from build123d import *

# Parameters (mm, degrees)
ESQUISSE1_W        = 39.37
ESQUISSE1_H        = 35.56
ESQUISSE1_R        = 1.65
BOSS_EXTRU_1_DEPTH = 2
CONG_2_R           = 5


with BuildPart() as part:
    # Esquisse1 → Boss.-Extru.1 (new body)
    with BuildSketch(Plane(origin=(0, 0, 0), x_dir=(1, 0, 0), z_dir=(0, 1, 0))):
        Rectangle(ESQUISSE1_W, ESQUISSE1_H)
        with Locations((-15.855, 13.97)):
            Circle(ESQUISSE1_R, mode=Mode.SUBTRACT)
        with Locations((15.855, 13.97)):
            Circle(ESQUISSE1_R, mode=Mode.SUBTRACT)
        with Locations((-15.855, -13.97)):
            Circle(ESQUISSE1_R, mode=Mode.SUBTRACT)
        with Locations((15.855, -13.97)):
            Circle(ESQUISSE1_R, mode=Mode.SUBTRACT)
    extrude(amount=BOSS_EXTRU_1_DEPTH)

    # Congé2
    cong_2_edges = [part.edges().sort_by_distance(p)[0] for p in [
        (19.685, 1, 17.78),
        (-19.685, 1, 17.78),
        (-19.685, 1, -17.78),
        (19.685, 1, -17.78),
    ]]
    fillet(cong_2_edges, radius=CONG_2_R)


solid = part.part
The listing builds one solid part. Answer for the finished solid, in the listing's coordinates (mm). Give positions to 0.01 mm unless a question says otherwise; leave off trailing zeros. Order: outer loops, then holes, each group sorted by start corner. A loop starts at its lowest first (then second) coordinate and runs counter-clockwise, first axis right, second up. Notation, with made-up numbers: (15, 69) - (42, 69) arc R28 ccw to (42, 93) - close; hole circle Ø3 at (40.5, 49.5). An arc over 180 degrees is marked (long way). Use one line per item in the form item = value.
1) The mould has two halves that part along Z. Classify faces 1 (the cylindrical face through (18.181, 1.014, -16.354)), 2 (the flat face through (0, 2, 0)), 3 (the cylindrical face through (-16.21, 0.99, -12.36)): released by +Z, released by -Z, zero draft, split by the parting line, or undercut.
Verdict:
face_1 = released by -Z
face_2 = zero draft
face_3 = undercut
2) Find section A-A on y = 0.3. Determine the outline of the cut face in (x, z) (3 decimals), and give its area (3 significant figures).
Verdict:
outline = (-19.685, -12.78) arc R5 ccw to (-14.685, -17.78) - (14.685, -17.78) arc R5 ccw to (19.685, -12.78) - (19.685, 12.78) arc R5 ccw to (14.685, 17.78) - (-14.685, 17.78) arc R5 ccw to (-19.685, 12.78) - close; hole circle Ø3.3 at (-15.855, -13.97); hole circle Ø3.3 at (-15.855, 13.97); hole circle Ø3.3 at (15.855, -13.97); hole circle Ø3.3 at (15.855, 13.97)
area = 1,340 mm^2
3) This flat-tipped pin is pushed along its axis until it touches: pin 1 (3 mm diameter, centred on x = 15.855, z = -13.97, fed in from -Y). Where does it stop, or does it pass through?
Verdict:
pin_1 = through
4) Find section C-C on x = -16. Determine the outline of the cut face in (y, z).
Verdict:
outline = (0, -17.6) - (2, -17.6) - (2, -15.61) - (0, -15.61) - close; (0, -12.33) - (2, -12.33) - (2, 12.33) - (0, 12.33) - close; (0, 15.61) - (2, 15.61) - (2, 17.6) - (0, 17.6) - close
5) Find section B-B on z = -15. Determine the outline of the cut face in (x, y), and give its area (3 significant figures).
Verdict:
outline = (-19.17, 0) - (-17.14, 0) - (-17.14, 2) - (-19.17, 2) - close; (-14.57, 0) - (14.57, 0) - (14.57, 2) - (-14.57, 2) - close; (17.14, 0) - (19.17, 0) - (19.17, 2) - (17.14, 2) - close
area = 66.3 mm^2
6) Consider probe 1 along Z at (x, y) = (-16, 1.7); probe 2 along X at (y, z) = (0.75, -13); probe 3 along Z at (x, y) = (15.5, 1.25). Determine where each line is inside the solid, lowest interval first. Write a range as [from, to].
Verdict:
probe_1 = [-17.6, -15.61], [-12.33, 12.33], [15.61, 17.6]
probe_2 = [-19.68, -17.19], [-14.52, 14.52], [17.19, 19.68]
probe_3 = [-17.71, -15.58], [-12.36, 12.36], [15.58, 17.71]
